```python
from build123d import *

# Parameters (mm, degrees)
SKETCH1_R           = 7.25
BOSS_EXTRUDE1_DEPTH = 1
BOSS_EXTRUDE2_DEPTH = 5
SKETCH3_R           = 4
CUT_EXTRUDE1_DEPTH  = 12.879604371


with BuildPart() as part:
    # Sketch1 → Boss-Extrude1 (new body)
    with BuildSketch(Plane(origin=(0, 0, 0), x_dir=(1, 0, 0), z_dir=(0, 1, 0))):
        with Locations(Location((0, 0, 0), (0, 0, 270))):
            Circle(SKETCH1_R)
    extrude(amount=BOSS_EXTRUDE1_DEPTH)

    # Sketch2 → Boss-Extrude2 (add)
    with BuildSketch(Plane(origin=(0, 1, 0), x_dir=(1, 0, 0), z_dir=(0, 1, 0))):
        with BuildLine():
            ThreePointArc((3.749975746, 6.204851482), (3.625, 6.278684177), (3.498571137, 6.35))
            Line((3.498571137, 6.35), (-3.498571137, 6.35))
            ThreePointArc((-3.498571137, 6.35), (-3.625, 6.278684177), (-3.749975746, 6.204851482))
            Line((-3.749975746, 6.204851482), (-7.248546882, 0.145148518))
            ThreePointArc((-7.248546882, 0.145148518), (-7.25, 0), (-7.248546882, -0.145148518))
            Line((-7.248546882, -0.145148518), (-3.749975746, -6.204851482))
            ThreePointArc((-3.749975746, -6.204851482), (-3.625, -6.278684177), (-3.498571137, -6.35))
            Line((-3.498571137, -6.35), (3.498571137, -6.35))
            ThreePointArc((3.498571137, -6.35), (3.625, -6.278684177), (3.749975746, -6.204851482))
            Line((3.749975746, -6.204851482), (7.248546882, -0.145148518))
            ThreePointArc((7.248546882, -0.145148518), (7.249636712, -0.072577896), (7.25, 0))
            ThreePointArc((7.25, 0), (7.249636712, 0.072577896), (7.248546882, 0.145148518))
            Line((7.248546882, 0.145148518), (3.749975746, 6.204851482))
        make_face()
    extrude(amount=BOSS_EXTRUDE2_DEPTH)

    # Sketch3 → Cut-Extrude1 (cut, through all)
    with BuildSketch(Plane(origin=(0, 6, 0), x_dir=(1, 0, 0), z_dir=(0, 1, 0))):
        with Locations(Location((0, 0, 0), (0, 0, 270))):
            Circle(SKETCH3_R)
    extrude(amount=-CUT_EXTRUDE1_DEPTH, mode=Mode.SUBTRACT)


solid = part.part
```
Verification items for the finished model (mm, model axes). A direction names the side the tool comes from. Give positions to 0.01 mm unless a question says otherwise; leave off trailing zeros. Order: outer loops, then holes, each group sorted by start corner. A loop starts at its lowest first (then second) coordinate and runs counter-clockwise, first axis right, second up. Notation, with made-up numbers: M 38,64.5 L 96,64.5 A16 ccw 96,74.5 Z; hole C 33.25,48 d3. An arc over 180 degrees is marked long. Return JSON: item names as keys, results as strings. Group by question number.
1) Go/stop test with flat-tipped pins: pin 1 Ø2.5 at (x, y) = (-1, 4.5) entering from +Z; pin 2 Ø1 at (x, z) = (1.5, 7) entering from +Y; pin 3 Ø1.5 at (y, z) = (1, 3.5) entering from -X. Record where each tip stops, or that it passes through.
2) Scan lines: line 1 (Y direction, x = 6, z = -3.5); line 2 (Z direction, x = -3, y = 3.95); line 3 (X direction, y = 1.6, z = 2.75). Record each from-to range of solid material in increasing order.
3) Section check B-B on y = 2.05. Record the cut outline in (x, z), and give its area (3 significant figures).
4) Access from +Z, -Z, +X, -X, +Y, -Y to the whole of each face (thin tool, end or side, straight path). Record for faces 1 (the face through (5.524, 3.465, -3.133)), 2 (the face through (-5.475, 3.465, -3.217)), 3 (the face through (-6, 1, 3)).
5) Mould release check, pull along Z, two halves, no side actions. Record for faces 4 (the face through (-3.905, 3.042, -0.867)), 5 (the face through (0, 3, -6.35)), 6 (the face through (6, 1, 3)): pulls with the +Z half, pulls with the -Z half, needs draft (parallel to the pull), parting line crosses it, or undercut.
6) Section check D-D on x = -5.75. Record the cut outline in (y, z).
7) Section check A-A on x = 0. Record the cut outline in (y, z), and give its area (3 significant figures).
8) Section check C-C on z = 0.5. Record the cut outline in (x, y).
Answer block:
{
 "1": {"pin 1": "stops at z = 6.35", "pin 2": "stops at y = 1", "pin 3": "stops at x = -6.71"},
 "2": {"line 1": "y = 0 to 1", "line 2": "z = -6.35 to -2.65, 2.65 to 6.35", "line 3": "x = -5.74 to -2.9, 2.9 to 5.74"},
 "3": {"outline": "M -7.25,-0.15 L -3.75,-6.2 A7.25 ccw -3.5,-6.35 L 3.5,-6.35 A7.25 ccw 3.75,-6.2 L 7.25,-0.15 A7.25 ccw 7.25,0.15 L 3.75,6.2 A7.25 ccw 3.5,6.35 L -3.5,6.35 A7.25 ccw -3.75,6.2 L -7.25,0.15 A7.25 ccw Z; hole C 0,0 d8", "area": "89.3 mm^2"},
 "4": {"face 1": "-Z, +X, +Y", "face 2": "-Z, -X, +Y", "face 3": "+Z, -X, +Y"},
 "5": {"face 4": "undercut", "face 5": "pulls with the -Z half", "face 6": "needs draft"},
 "6": {"outline": "M 0,-4.42 L 1,-4.42 L 1,-2.74 L 6,-2.74 L 6,2.74 L 1,2.74 L 1,4.42 L 0,4.42 Z"},
 "7": {"outline": "M 0,-7.25 L 1,-7.25 L 1,-6.35 L 6,-6.35 L 6,-4 L 0,-4 Z; M 0,4 L 6,4 L 6,6.35 L 1,6.35 L 1,7.25 L 0,7.25 Z", "area": "30.0 mm^2"},
 "8": {"outline": "M -7.23,0 L -3.97,0 L -3.97,6 L -7.04,6 L -7.04,1 L -7.23,1 Z; M 3.97,0 L 7.23,0 L 7.23,1 L 7.04,1 L 7.04,6 L 3.97,6 Z"}
}
